Read the model definition and answer for the solid it produces. Units are mm, in the model's axes. Face numbers are marked on the shaded views. Round coordinates to 2 decimals unless told otherwise and drop trailing zeros. Order: outer loops, then holes, each group sorted by start corner. A loop starts at its lowest first (then second) coordinate and runs counter-clockwise, first axis right, second up. Notation, with made-up numbers: M -28,-19.5 L 19,-19.5 A12 ccw 19,-9.5 Z; hole C 78,-3.75 d1. An arc over 180 degrees is marked long. Use one line per item in the form item = value. Start each with the question number.
from build123d import *

# Parameters (mm, degrees)
LOFT1_OUTLINE_W     = 45.5
LOFT1_OUTLINE_H     = 128.5
LOFT1_DEPTH         = 3
LOFT1_DRAFT         = 45
LOFT2_START         = -6
LOFT2_OUTLINE_W     = 51.5
LOFT2_OUTLINE_H     = 134.5
LOFT2_DEPTH         = 3
SKETCH4_W           = 42.5
SKETCH4_H           = 3
BOSS_EXTRUDE1_DEPTH = 44
SKETCH5_W           = 11.5
SKETCH5_H           = 10
CUT_EXTRUDE1_DEPTH  = 45.5
SKETCH6_W           = 37.00940911
SKETCH6_H           = 2.5
BOSS_EXTRUDE2_DEPTH = 12
SKETCH7_W           = 3.2
SKETCH7_H           = 10.2
CUT_EXTRUDE2_DEPTH  = 3


# Read off the part's stored shape, not the designer's step: Loft1, Loft2
with BuildPart() as part:
    # Loft1 outline → Loft1 (with draft: the straight prism first)
    with BuildSketch(Plane(origin=(0, 0, 0), x_dir=(1, 0, 0), z_dir=(0, 1, 0))):
        Rectangle(LOFT1_OUTLINE_W, LOFT1_OUTLINE_H)
    extrude(amount=-LOFT1_DEPTH)
    # Loft1: the draft: its side faces are tilted about the plane it starts from
    loft1_sides = [part.faces().sort_by_distance(p)[0] for p in [
        (22.75, -1.5, 0),
        (0, -1.5, -64.25),
        (-22.75, -1.5, 0),
        (0, -1.5, 64.25),
    ]]
    draft(loft1_sides, Plane(origin=(0, 0, 0), x_dir=(1, 0, 0), z_dir=(0, 1, 0)), LOFT1_DRAFT)

    # Loft2 outline → Loft2 (add)
    with BuildSketch(Plane(origin=(0, 0, 0), x_dir=(1, 0, 0), z_dir=(0, 1, 0)).offset(LOFT2_START)):
        Rectangle(LOFT2_OUTLINE_W, LOFT2_OUTLINE_H)
    extrude(amount=LOFT2_DEPTH)

    # Sketch4 → Boss-Extrude1 (add)
    with BuildSketch(Plane(origin=(0, 0, 0), x_dir=(1, 0, 0), z_dir=(0, 1, 0))):
        with Locations((0, -62.75)):
            Rectangle(SKETCH4_W, SKETCH4_H)
    extrude(amount=BOSS_EXTRUDE1_DEPTH)

    # Sketch5 → Cut-Extrude1 (cut)
    with BuildSketch(Plane.XY.offset(64.25)):
        with Locations((-2, 5)):
            Rectangle(SKETCH5_W, SKETCH5_H)
    extrude(amount=-CUT_EXTRUDE1_DEPTH, mode=Mode.SUBTRACT)

    # Sketch6 → Boss-Extrude2 (add)
    with BuildSketch(Plane(origin=(0, 0, 0), x_dir=(1, 0, 0), z_dir=(0, 1, 0))):
        with Locations((0, 1)):
            Rectangle(SKETCH6_W, SKETCH6_H)
    extrude(amount=BOSS_EXTRUDE2_DEPTH)

    # Sketch7 → Cut-Extrude2 (cut)
    with BuildSketch(Plane(origin=(0, 0, 0), x_dir=(1, 0, 0), z_dir=(0, 1, 0))):
        with Locations((-21.15, 47.15)):
            Rectangle(SKETCH7_W, SKETCH7_H)
        with Locations((21.15, 47.15)):
            Rectangle(SKETCH7_W, SKETCH7_H)
        with Locations((-21.15, -47.15)):
            Rectangle(SKETCH7_W, SKETCH7_H)
        with Locations((21.15, -47.15)):
            Rectangle(SKETCH7_W, SKETCH7_H)
    extrude(amount=-CUT_EXTRUDE2_DEPTH, mode=Mode.SUBTRACT)


solid = part.part
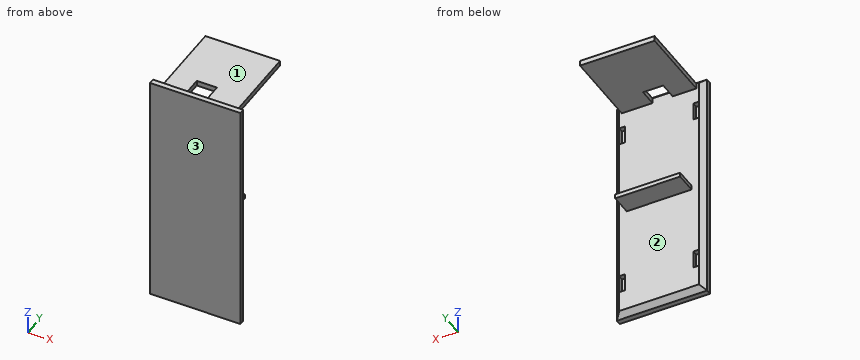
Item 1: Find the intervals of material crossed by L1, parallel to Z at x = 8.5, y = 7; L2, parallel to Y at x = -15, z = -41.5; L3, parallel to Z at x = -13, y = 18, in increasing order. Write a range as [from, to].
Item 2: Section D-D (x = -13) is taken. Write down the section's boundary in (y, z), and give its area (3 significant figures).
Item 3: Section A-A (y = 2.5) is taken. Write down the section's boundary in (x, z), and give its area (3 significant figures).
Item 4: For a pull along Z with two mould halves and no side action, classify the marked faces 1, 2 and 3 as pulls with the +Z half, pulls with the -Z half, needs draft (parallel to the pull), parting line crosses it, or undercut.
Item 5: Section B-B (x = -5.5) is taken. Write down the section's boundary in (y, z), and give its area (3 significant figures).
Item 6: Section C-C (z = -50.5) is taken. Write down the section's boundary in (x, y), and give its area (3 significant figures).
Item 7: Given P1, Ø1, axis at x = 17.5, y = 25, coming from the -Z side; P2, Ø0.9, axis at y = -2, z = -49.5, coming from the -X side; P3, Ø2, axis at x = -7, z = 45, coming from the +Y side; P4, Ø3.5, axis at y = -1.5, z = -49.5, coming from the +X side, each flat-ended and moving along its own axis, determine where each tip first touches the part or whether it passes through.
The answers:
q1.L1 = [-2.25, 0.25], [61.25, 64.25]
q1.L2 = [-6, 0]
q1.L3 = [61.25, 64.25]
q2.outline = M -6,-67.25 L -3,-67.25 L 0,-64.25 L 0,-2.25 L 12,-2.25 L 12,0.25 L 0,0.25 L 0,61.25 L 44,61.25 L 44,64.25 L 0,64.25 L -3,67.25 L -6,67.25 Z
q2.area = 960 mm²
q3.outline = M -21.25,61.25 L -7.75,61.25 L -7.75,64.25 L -21.25,64.25 Z; M -18.5,-2.25 L 18.5,-2.25 L 18.5,0.25 L -18.5,0.25 Z; M 3.75,61.25 L 21.25,61.25 L 21.25,64.25 L 3.75,64.25 Z
q3.area = 186 mm²
q4.face_1 = pulls with the +Z half
q4.face_2 = undercut
q4.face_3 = needs draft
q5.outline = M -6,-67.25 L -3,-67.25 L 0,-64.25 L 0,-2.25 L 12,-2.25 L 12,0.25 L 0,0.25 L 0,64.25 L -3,67.25 L -6,67.25 Z; M 10,61.25 L 44,61.25 L 44,64.25 L 10,64.25 Z
q5.area = 930 mm²
q6.outline = M -25.75,-6 L 25.75,-6 L 25.75,-3 L 22.75,0 L 22.75,-3 L 19.55,-3 L 19.55,0 L -19.55,0 L -19.55,-3 L -22.75,-3 L -22.75,0 L -25.75,-3 Z
q6.area = 281 mm²
q7.P1 = 61.25
q7.P2 = -25.2
q7.P3 = 0
q7.P4 = 25.75
